Solid Edge part; units mm, degrees
sketch "Sketch1" plane through (0, 0, 0) normal (0, 0, 1) x (1, 0, 0)
  circle A0 centre (0, 0) radius 9.525
extrude "Protrusion1" add sketch "Sketch1" along normal blind 7.9248
sketch "Sketch2" plane through (0, 0, 0) normal (0, 0, -1) x (0, 1, 0)
  circle A0 centre (0, 0) radius 6.35
extrude "Protrusion2" add sketch "Sketch2" along normal blind 19.05
sketch "Sketch3" plane through (0, 0, -19.05) normal (0, 0, -1) x (0, 1, 0)
  circle A0 centre (0, 0) radius 4.7625
extrude "Protrusion3" add sketch "Sketch3" along normal blind 15.875
sketch "Sketch4" plane through (0, 0, 7.9248) normal (0, 0, 1) x (0, 1, 0)
  line L0 (-3.175, 1.7461) -> (0, 3.8287)
  line L1 (-3.175, -2.051) -> (-3.175, 1.7461)
  line L2 (-3.175, -2.051) -> (0, -3.8287)
  line L3 (3.175, -2.051) -> (0, -3.8287)
  line L4 (3.175, -2.051) -> (3.175, 1.7461)
  line L5 (3.175, 1.7461) -> (0, 3.8287)
extrude "Cutout1" cut sketch "Sketch4" against normal blind 3.9624
chamfer "Chamfer1" distance 0.7874 angle 45 1 edges at (0, -4.7625, -34.925)
properties part number "153181"
Geometry check sheet. Reference: the model listing, model coordinates, mm. A direction names the side the tool comes from. Give positions to 0.01 mm unless a question says otherwise; leave off trailing zeros. Order: outer loops, then holes, each group sorted by start corner. A loop starts at its lowest first (then second) coordinate and runs counter-clockwise, first axis right, second up.
1. Gauge pin test, flat ends, axial feed: pin 1 Ø1 at (x, z) = (1.5, 0.5) entering from -Y; pin 2 Ø10 at (y, z) = (-2, -27.5) entering from -X; pin 3 Ø4 at (y, z) = (3, 0) entering from -X. Record the tip position at first contact, or that the pin passes through.
2. Section check B-B, the plane z = -10. Enter the section's corners in (x, y), and give its area (3 significant figures).
3. Section check D-D, the plane z = -21.5. Enter the section's corners in (x, y) (1 decimal), and give its area (3 significant figures).
4. Thickness scan on L1, parallel to Z at x = -1, y = 7.25; L2, parallel to Z at x = -3.25, y = 0.5 (3 decimals); L3, parallel to X at y = 1.75, z = 6.5. Record the ranges inside material, lowest first.
5. Section check C-C, the plane y = -5.75. Enter the section's corners in (x, z), and give its area (3 significant figures).
6. Access from +Z, -Z, +X, -X, +Y, -Y to the whole of each face (thin tool, end or side, straight path). Record for faces 1 (the face through (-1, 5, -19.05)), 2 (the face through (-7.559, 5.796, 3.907)), 3 (the face through (0, 3.175, 6)).
7. Release check for a two-part mould opening along Y. For faces 4 (the face through (-2.773, 1.61, 5.971)), 5 (the face through (2.9, -3.78, -26.49)), 6 (the face through (0, 0, -34.925)) record: pulls with the +Y half, pulls with the -Y half, needs draft (parallel to the pull), parting line crosses it, or undercut.
Values follow:
1. pin 1: stops at y = -9.47
1. pin 2: stops at x = -4.76
1. pin 3: stops at x = -9.47
2. outline: circle Ø12.7 at (0, 0)
2. area: 127 mm2
3. outline: circle Ø9.5 at (0, 0)
3. area: 71.3 mm2
4. L1: z = 0 to 7.92
4. L2: z = -34.925 to 3.962
4. L3: x = -9.36 to -2.68, 2.85 to 9.36
5. outline: (-7.59, 0) - (-2.69, 0) - (-2.69, -19.05) - (2.69, -19.05) - (2.69, 0) - (7.59, 0) - (7.59, 7.92) - (-7.59, 7.92) - close
5. area: 223 mm2
6. face 1: -Z
6. face 2: +Z, -Z
6. face 3: +Z
7. face 4: undercut
7. face 5: parting line crosses it
7. face 6: needs draft
